Could you check a few things on this model? Use its own coordinates, in mm. A direction names the side the tool comes from. Round coordinates to 2 decimals unless told otherwise and drop trailing zeros. Write each loop counter-clockwise with the first axis right and the second up, starting at its lowest first coordinate (ties: lowest second). Pieces come first, ordered by that corner, then holes. Notation, with made-up numbers: (17.25, -29) -> (68.25, -29) arc R18 ccw to (68.25, -12) -> close; hole circle Ø10 at (5, -2.5). An arc over 180 degrees is marked (long way). Return JSON: item names as keys, results as strings.
from build123d import *

# Parameters (mm, degrees)
F0_W     = 104
F0_H     = 80
F0_R     = 2.75
F0_R_2   = 2
F0_R_3   = 18.5
F1_DEPTH = 12
F2_R     = 4.5
F3_DEPTH = 5


with BuildPart() as f1:
    # F0 (on Front) → F1 (new body)
    with BuildSketch(Plane.XZ):
        with Locations((52, 40)):
            Rectangle(F0_W, F0_H)
        with Locations((6, 15)):
            Circle(F0_R, mode=Mode.SUBTRACT)
        with Locations((27, 15)):
            Circle(F0_R_2, mode=Mode.SUBTRACT)
        with Locations((77, 15)):
            Circle(F0_R_2, mode=Mode.SUBTRACT)
        with Locations((98, 15)):
            Circle(F0_R, mode=Mode.SUBTRACT)
        with Locations((6, 65)):
            Circle(F0_R, mode=Mode.SUBTRACT)
        with Locations((27, 65)):
            Circle(F0_R_2, mode=Mode.SUBTRACT)
        with Locations((52, 40)):
            Circle(F0_R_3, mode=Mode.SUBTRACT)
        with Locations((77, 65)):
            Circle(F0_R_2, mode=Mode.SUBTRACT)
        with Locations((98, 65)):
            Circle(F0_R, mode=Mode.SUBTRACT)
    extrude(amount=F1_DEPTH)

    # F2 (on face) → F3 (cut)
    with BuildSketch(Plane.XZ.offset(12)):
        with Locations((6, 65)):
            Circle(F2_R)
        with Locations((98, 65)):
            Circle(F2_R)
        with Locations((98, 15)):
            Circle(F2_R)
        with Locations((6, 15)):
            Circle(F2_R)
    extrude(amount=-F3_DEPTH, mode=Mode.SUBTRACT)


solid = f1.part
1) I want a section at D-D, the plane x = 66.5. Please give me the cut outline in (y, z), and give its area (3 significant figures).
Return value:
{"outline": "(-12, 0) -> (0, 0) -> (0, 28.51) -> (-12, 28.51) -> close; (-12, 51.49) -> (0, 51.49) -> (0, 80) -> (-12, 80) -> close", "area": "684 mm²"}
2) For faces 1 (the face through (95.253, -3.451, 15.121)), 2 (the face through (9, -7, 65)), which set-ups out of +Z, -Z, +X, -X, +Y, -Y let a thin tool reach every point of the face, with its end or its side?
Return value:
{"face 1": "+Y, -Y", "face 2": "-Y"}
3) If I drill on probe 1 along Z at (x, y) = (6, -3.25); probe 2 along Z at (x, y) = (77, -8.25); probe 3 along Z at (x, y) = (52, -3.75), over which ranges is the centre line in solid material (lowest first)? Write a range as [from, to].
Return value:
{"probe 1": "[0, 12.25], [17.75, 62.25], [67.75, 80]", "probe 2": "[0, 13], [17, 63], [67, 80]", "probe 3": "[0, 21.5], [58.5, 80]"}
4) Thinking about a two-plate mould opening in Z: for faces 3 (the face through (51, -6, 80)), 4 (the face through (8.419, -9.535, 18.794)), 5 (the face through (63, -12, 58)), which applies, pulls with the +Z half, pulls with the -Z half, needs draft (parallel to the pull), parting line crosses it, or undercut?
Return value:
{"face 3": "pulls with the +Z half", "face 4": "undercut", "face 5": "needs draft"}
5) I want a section at B-B, the plane z = 40. Please give me the cut outline in (x, y).
Return value:
{"outline": "(0, -12) -> (33.5, -12) -> (33.5, 0) -> (0, 0) -> close; (70.5, -12) -> (104, -12) -> (104, 0) -> (70.5, 0) -> close"}
6) I want a section at A-A, the plane x = 77. Please give me the cut outline in (y, z).
Return value:
{"outline": "(-12, 0) -> (0, 0) -> (0, 13) -> (-12, 13) -> close; (-12, 17) -> (0, 17) -> (0, 63) -> (-12, 63) -> close; (-12, 67) -> (0, 67) -> (0, 80) -> (-12, 80) -> close"}
7) I want a section at C-C, the plane y = -10. Count the separate pieces of the cut face and the enclosed holes in it, and give its area (3 significant figures).
Return value:
{"separate pieces": "1", "enclosed holes": "9", "area": "6,940 mm²"}
8) Will these pins go through, and if not, where does the flat tip stop? pin 1 Ø7 at (x, z) = (98, 15) entering from -Y; pin 2 Ø3.5 at (x, z) = (27, 15) entering from -Y.
Return value:
{"pin 1": "y = -7", "pin 2": "through"}
